The listing builds one solid part. Answer for the finished solid, in the listing's coordinates (mm). Face numbers are marked on the shaded views. A direction names the side the tool comes from. Round coordinates to 2 decimals unless told otherwise and drop trailing zeros. Write each loop counter-clockwise with the first axis right and the second up, starting at its lowest first coordinate (ties: lowest second). Pieces come first, ordered by that corner, then holes. Notation, with made-up numbers: (66, 18) - (123, 18) arc R27 cw to (123, 53) - close; hole circle Ø9 at (-6, -14.75). An arc over 180 degrees is marked (long way). Return JSON: item names as keys, results as strings. Group by question number.
(1) Section C-C, the plane y = 15.25 is taken. Write down the section's boundary in (x, z), then the cut area to 3 significant figures.
(2) Section B-B, the plane z = 0 is taken. Write down the section's boundary in (x, y).
(3) Find the intervals of material crossed by line 1 along X through (y, z) = (8.25, -17); line 2 along X through (y, z) = (15, 0); line 3 along Y through (x, z) = (0, -24.5), in increasing order. Write a range as [from, to].
(4) Which of the six approach directions +Z, -Z, +X, -X, +Y, -Y give full straight-line access (tool end or side, diameter ignored) to the marked faces 1, 2 and 3?
(5) Determine the mould class of the marked faces 4, 5, 6 and 7 for opening direction X: +X half, -X half, draft (parallel to the pull), parting line (faces both ways), or undercut.
(6) Each of these flat-tipped pins is pushed along its axis until it touches: pin 1 (6.5 mm diameter, centred on x = 0, z = -6, fed in from +Y); pin 2 (7.5 mm diameter, centred on y = 15, z = -13.5, fed in from +X); pin 3 (1.5 mm diameter, centred on y = 16.5, z = -15, fed in from -X). Where does it stop, or does it pass through?
(7) Section D-D, the plane y = 4.25 is taken. Write down the section's boundary in (x, z), then the cut area to 3 significant figures.
(8) Section A-A, the plane x = 0 is taken. Write down the section's boundary in (y, z), then the cut area to 3 significant figures.
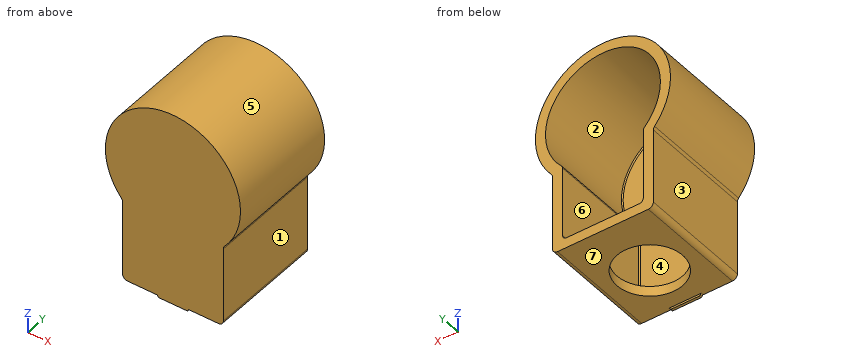
```python
from build123d import *

# Parameters (mm, degrees)
BOSS_EXTRUDE1_DEPTH = 20.574
BOSS_EXTRUDE2_START = 2
BOSS_EXTRUDE2_DEPTH = 2
SKETCH3_R           = 6.5
CUT_EXTRUDE1_DEPTH  = 45.007669834
FILLET1_R           = 1
SKETCH4_W           = 6
SKETCH4_H           = 0.5
BOSS_EXTRUDE3_DEPTH = 0.4
FILLET2_START       = -3
FILLET2_DEPTH       = 2
FILLET2_START_2     = -2
FILLET2_2_DEPTH     = 0.5
FILLET3_R           = 0.8
CHAMFER1_SIZE       = 0.2


with BuildPart() as part:
    # Sketch1 → Boss-Extrude1 (new body)
    with BuildSketch(Plane(origin=(0, 0, 0), x_dir=(1, 0, 0), z_dir=(0, 1, 0))):
        with BuildLine():
            Line((10, 8.919641248), (10, 25.121576202))
            Line((10, 25.121576202), (-10, 25.121576202))
            Line((-10, 25.121576202), (-10, 8.919641248))
            ThreePointArc((-10, 8.919641248), (0, -13.4), (10, 8.919641248))
        make_face()
        with BuildLine():
            Line((-8, 23.121576202), (-8, 8.121576202))
            ThreePointArc((-8, 8.121576202), (0, -11.4), (8, 8.121576202))
            Line((8, 8.121576202), (8, 23.121576202))
            Line((8, 23.121576202), (-8, 23.121576202))
        make_face(mode=Mode.SUBTRACT)
    extrude(amount=BOSS_EXTRUDE1_DEPTH)

    # Sketch2 → Boss-Extrude2 (add)
    with BuildSketch(Plane.XZ.offset(BOSS_EXTRUDE2_START)):
        with BuildLine():
            Line((10, -8.919641248), (10, -25.121576202))
            Line((10, -25.121576202), (-10, -25.121576202))
            Line((-10, -25.121576202), (-10, -8.919641248))
            ThreePointArc((-10, -8.919641248), (0, 13.4), (10, -8.919641248))
        make_face()
    extrude(amount=-BOSS_EXTRUDE2_DEPTH)

    # Sketch3 → Cut-Extrude1 (cut, through all)
    with BuildSketch(Plane.XY.offset(-23.121576202)):
        with Locations((0, 8)):
            Circle(SKETCH3_R)
    extrude(amount=-CUT_EXTRUDE1_DEPTH, mode=Mode.SUBTRACT)

    # Fillet1
    fillet1_edges = [part.edges().sort_by_distance(p)[0] for p in [
        (-10, 9.287, -8.919641248),
        (-10, 9.287, -25.121576202),
        (10, 9.287, -25.121576202),
        (10, 9.287, -8.919641248),
    ]]
    fillet(fillet1_edges, radius=FILLET1_R)

    # Sketch4 → Boss-Extrude3 (add)
    with BuildSketch(Plane(origin=(0, 0, -25.121576202), x_dir=(-1, 0, 0), z_dir=(0, 0, -1))):
        with Locations((0, -1.75)):
            Rectangle(SKETCH4_W, SKETCH4_H)
    extrude(amount=BOSS_EXTRUDE3_DEPTH)

    # Fillet2: read off the stored shape, not the designer's step
    # Fillet2 outline → Fillet2 (cut)
    with BuildSketch(Plane(origin=(0, 0, 0), x_dir=(1, 0, 0), z_dir=(0, 1, 0)).offset(FILLET2_START)):
        with BuildLine():
            ThreePointArc((-3, 25.321576202), (-2.941421356, 25.462997558), (-2.8, 25.521576202))
            Line((-2.8, 25.521576202), (-3, 25.521576202))
            Line((-3, 25.521576202), (-3, 25.321576202))
        make_face()
        with BuildLine():
            Line((3, 25.521576202), (2.8, 25.521576202))
            ThreePointArc((2.8, 25.521576202), (2.941421356, 25.462997558), (3, 25.321576202))
            Line((3, 25.321576202), (3, 25.521576202))
        make_face()
    extrude(amount=FILLET2_DEPTH, mode=Mode.SUBTRACT)

    # Fillet2 2 outline → Fillet2 2 (add)
    with BuildSketch(Plane(origin=(0, 0, 0), x_dir=(1, 0, 0), z_dir=(0, 1, 0)).offset(FILLET2_START_2)):
        with BuildLine():
            Line((-3, 25.121576202), (-3, 25.321576202))
            ThreePointArc((-3, 25.321576202), (-3.058578644, 25.180154845), (-3.2, 25.121576202))
            Line((-3.2, 25.121576202), (-3, 25.121576202))
        make_face()
        with BuildLine():
            ThreePointArc((3.2, 25.121576202), (3.058578644, 25.180154845), (3, 25.321576202))
            Line((3, 25.321576202), (3, 25.121576202))
            Line((3, 25.121576202), (3.2, 25.121576202))
        make_face()
    extrude(amount=FILLET2_2_DEPTH)

    # Fillet3
    fillet3_edges = [part.edges().sort_by_distance(p)[0] for p in [
        (8, 10.287, -23.121576202),
        (-8, 10.287, -23.121576202),
        (-8, 10.287, -8.121576202),
        (8, 10.287, -8.121576202),
    ]]
    fillet(fillet3_edges, radius=FILLET3_R)

    # Chamfer1
    chamfer1_edges = [part.edges().sort_by_distance(p)[0] for p in [
        (8, 0, -15.385714136),
        (0, 0, -23.121576202),
        (-8, 0, -15.385714136),
        (0, 0, 11.4),
        (-7.765685425, 0, -22.887261627),
        (7.765685425, 0, -22.887261627),
        (8.057827734, 0, -8.151221315),
        (-8.057827734, 0, -8.151221315),
    ]]
    chamfer(chamfer1_edges, length=CHAMFER1_SIZE)


solid = part.part
```
Working result:
{
 "1": {"outline": "(-10.24, -8.65) arc R1 cw to (-10, -9.29) - (-10, -24.12) arc R1 ccw to (-9, -25.12) - (9, -25.12) arc R1 ccw to (10, -24.12) - (10, -9.29) arc R1 cw to (10.24, -8.65) arc R13.4 ccw (long way) to start; hole (-8.22, -7.9) arc R0.8 cw to (-8, -8.45) - (-8, -22.32) arc R0.8 ccw to (-7.2, -23.12) - (7.2, -23.12) arc R0.8 ccw to (8, -22.32) - (8, -8.45) arc R0.8 cw to (8.22, -7.9) arc R11.4 ccw (long way) to start", "area": "214 mm^2"},
 "2": {"outline": "(-13.4, -2) - (13.4, -2) - (13.4, 20.57) - (11.4, 20.57) - (11.4, 0.2) - (11.2, 0) - (-11.2, 0) - (-11.4, 0.2) - (-11.4, 20.57) - (-13.4, 20.57) - close"},
 "3": {"line 1": "x = [-10, -8], [8, 10]", "line 2": "x = [-13.4, -11.4], [11.4, 13.4]", "line 3": "y = [-2, 1.5], [14.5, 20.57]"},
 "4": {"face 1": "-Z, +X, +Y, -Y", "face 2": "+Y", "face 3": "-Z, -X, +Y, -Y"},
 "5": {"face 4": "undercut", "face 5": "parting line", "face 6": "undercut", "face 7": "draft"},
 "6": {"pin 1": "stops at y = 0", "pin 2": "stops at x = 10", "pin 3": "stops at x = -10"},
 "7": {"outline": "(-10.24, -8.65) arc R1 cw to (-10, -9.29) - (-10, -24.12) arc R1 ccw to (-9, -25.12) - (-5.31, -25.12) - (-5.31, -23.12) - (-7.2, -23.12) arc R0.8 cw to (-8, -22.32) - (-8, -8.45) arc R0.8 ccw to (-8.22, -7.9) arc R11.4 cw (long way) to (8.22, -7.9) arc R0.8 ccw to (8, -8.45) - (8, -22.32) arc R0.8 cw to (7.2, -23.12) - (5.31, -23.12) - (5.31, -25.12) - (9, -25.12) arc R1 ccw to (10, -24.12) - (10, -9.29) arc R1 cw to (10.24, -8.65) arc R13.4 ccw (long way) to start", "area": "193 mm^2"},
 "8": {"outline": "(-2, -25.52) - (-1.5, -25.52) - (-1.5, -25.12) - (1.5, -25.12) - (1.5, -23.12) - (0.2, -23.12) - (0, -22.92) - (0, 11.2) - (0.2, 11.4) - (20.57, 11.4) - (20.57, 13.4) - (-2, 13.4) - close; (14.5, -25.12) - (20.57, -25.12) - (20.57, -23.12) - (14.5, -23.12) - close", "area": "134 mm^2"}
}
